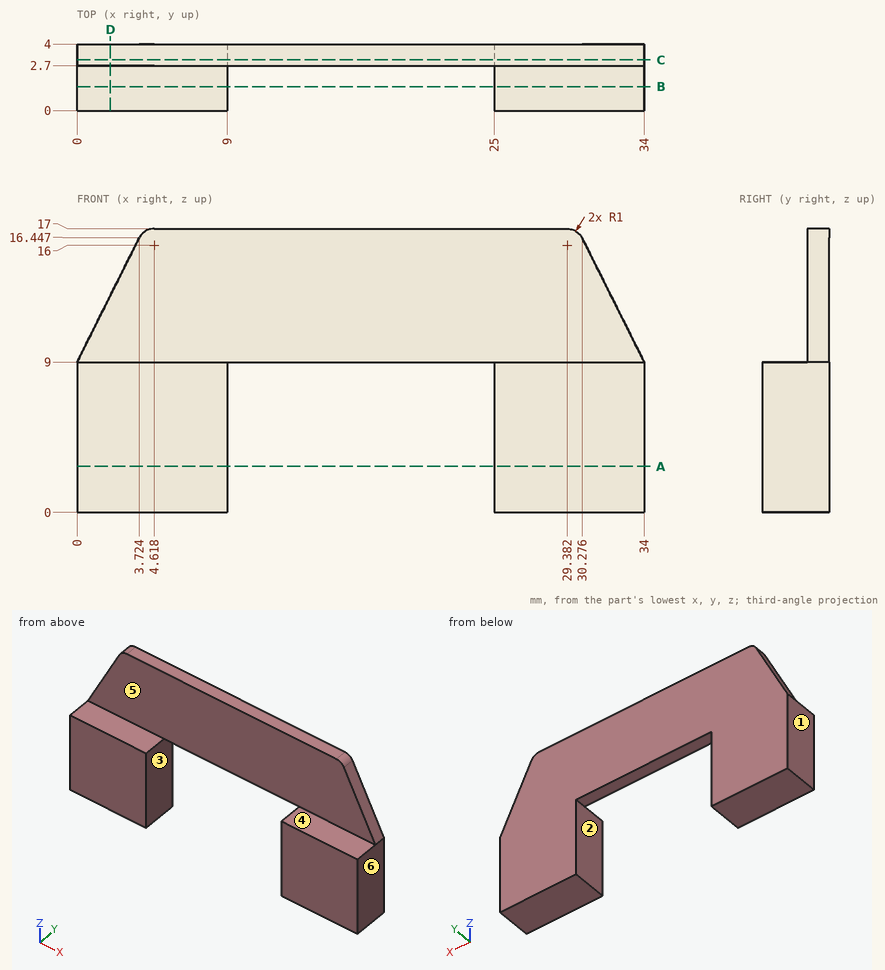
Geometry: see drawing. Coordinates: mm, zero at the bounding-box minimum. A direction names the side the tool comes from. Coordinates: 2 decimals unless noted, no trailing zeros. Write each loop counter-clockwise with the first axis right and the second up, starting at its lowest first coordinate (ties: lowest second). Pieces come first, ordered by that corner, then holes.
1) Mould query, pull axis X, two halves, no side actions, for the marked faces 1, 2, 3 and 4. Classes: pulls with the +X half, pulls with the -X half, needs draft (parallel to the pull), parting line crosses it, or undercut.
2) Pin query (flat end, axial travel): pin 1 Ø2.5 at (x, z) = (9.5, 14) entering from -Y; pin 2 Ø1.5 at (y, z) = (1, 4.5) entering from -X; pin 3 Ø1.4 at (x, y) = (5, 1) entering from +Z; pin 4 Ø0.6 at (x, y) = (19, 3.5) entering from -Z. Return the tip coordinate at first contact, or that it passes through.
3) Section D-D on x = 2. Output: boundary loops of the cut face in (y, z), and give its area (3 significant figures).
4) Material intervals for line 1 along X through (y, z) = (1.9, 3.75); line 2 along Z through (x, y) = (31, 2.55); line 3 along Y through (x, z) = (21.5, 12.5), sorted ascending.
5) Section A-A on z = 2.75. Output: boundary loops of the cut face in (x, y), and give its area (3 significant figures).
6) Set-up query: the marked faces 5 and 6. Return all of +Z, -Z, +X, -X, +Y, -Y with unobstructed straight access to the full face (end or side cutting, diameter ignored); none if empty.
7) Section B-B on y = 1.45. Output: boundary loops of the cut face in (x, z).
8) Section C-C on y = 3.05. Output: boundary loops of the cut face in (x, z), and give its area (3 significant figures).
Check result:
1. face 1: pulls with the -X half
1. face 2: undercut
1. face 3: undercut
1. face 4: needs draft
2. pin 1: stops at y = 2.7
2. pin 2: stops at x = 0
2. pin 3: stops at z = 9
2. pin 4: stops at z = 9
3. outline: (0, 0) - (4, 0) - (4, 13) - (2.7, 13) - (2.7, 9) - (0, 9) - close
3. area: 41.2 mm2
4. line 1: x = 0 to 9, 25 to 34
4. line 2: z = 0 to 9
4. line 3: y = 2.7 to 4
5. outline: (0, 0) - (9, 0) - (9, 4) - (0, 4) - close; (25, 0) - (34, 0) - (34, 4) - (25, 4) - close
5. area: 72.0 mm2
6. face 5: +Z, +X, -X, -Y
6. face 6: +Z, -Z, +X, +Y, -Y
7. outline: (0, 0) - (9, 0) - (9, 9) - (0, 9) - close; (25, 0) - (34, 0) - (34, 9) - (25, 9) - close
8. outline: (0, 0) - (9, 0) - (9, 9) - (25, 9) - (25, 0) - (34, 0) - (34, 9) - (30.28, 16.45) arc R1 ccw to (29.38, 17) - (4.62, 17) arc R1 ccw to (3.72, 16.45) - (0, 9) - close
8. area: 402 mm2
